The model under review builds one solid part; all positions refer to its coordinate system, in mm. A direction names the side the tool comes from. Coordinates: 2 decimals unless noted, no trailing zeros. Order: outer loops, then holes, each group sorted by start corner. A loop starts at its lowest first (then second) coordinate and runs counter-clockwise, first axis right, second up.
from build123d import *

# Parameters (mm, degrees)
F0_W     = 160
F0_H     = 90
F1_DEPTH = 40
F2_R     = 10
F3_T     = -2.5


with BuildPart() as f1:
    # F0 (on Top) → F1 (new body)
    with BuildSketch(Plane.XY):
        with Locations((-80, -45)):
            Rectangle(F0_W, F0_H)
    extrude(amount=F1_DEPTH)

    # F2
    f2_edges = [f1.edges().sort_by_distance(p)[0] for p in [
        (-160, -90, 20),
        (0, 0, 20),
        (0, -90, 20),
        (-160, 0, 20),
    ]]
    fillet(f2_edges, radius=F2_R)

    # F3
    f3_openings = [f1.faces().sort_by_distance(p)[0] for p in [
        (-80, -45, 40),
    ]]
    offset(amount=F3_T, openings=f3_openings)


solid = f1.part
(1) Tool access review of faces 4 (the face through (-2.85, -3.01, 20.28)), 5 (the face through (-2.5, -45, 21)): name each direction out of +Z, -Z, +X, -X, +Y, -Y from which nothing blocks a thin tool from reaching the whole face with its end or side.
(2) Insertion check: pin 1 Ø10 at (x, y) = (-132.5, -69) entering from +Z. The pin has a flat end and moves straight along its axis. Give the tip position at first contact, or say it passes through.
(3) Consider section A-A (z = 4.5). Give the boundary of the cut face in (x, y), then the cut area to 3 significant figures.
(4) The part is to be moulded in two halves that separate along Y. For faces 1 (the face through (-4.755, -85.361, 21.512)), 2 (the face through (0, -45, 20)), 3 (the face through (-81, -90, 20)), say which applies: +Y half, -Y half, draft (parallel to the pull), parting line (faces both ways), or undercut.
(5) Consider section B-B (x = -97.5). Give the boundary of the cut face in (y, z), then the cut area to 4 significant figures.
(6) Wall thickness on line 1 (X direction, y = -65, z = 29.5); line 2 (Y direction, x = -48, z = 28.5); line 3 (Z direction, x = -30.5, y = -73.5): over which ranges is each line inside the solid? List them lowest first.
(7) Consider section C-C (y = -50). Give the boundary of the cut face in (x, z).
Findings:
1. face 4: +Z, -Z, +X, +Y
1. face 5: +Z
2. pin 1: stops at z = 2.5
3. outline: (-160, -80) arc R10 ccw to (-150, -90) - (-10, -90) arc R10 ccw to (0, -80) - (0, -10) arc R10 ccw to (-10, 0) - (-150, 0) arc R10 ccw to (-160, -10) - close; hole (-157.5, -80) arc R7.5 ccw to (-150, -87.5) - (-10, -87.5) arc R7.5 ccw to (-2.5, -80) - (-2.5, -10) arc R7.5 ccw to (-10, -2.5) - (-150, -2.5) arc R7.5 ccw to (-157.5, -10) - close
3. area: 1,190 mm2
4. face 1: undercut
4. face 2: draft
4. face 3: -Y half
5. outline: (-90, 0) - (0, 0) - (0, 40) - (-2.5, 40) - (-2.5, 2.5) - (-87.5, 2.5) - (-87.5, 40) - (-90, 40) - close
5. area: 412.5 mm2
6. line 1: x = -160 to -157.5, -2.5 to 0
6. line 2: y = -90 to -87.5, -2.5 to 0
6. line 3: z = 0 to 2.5
7. outline: (-160, 0) - (0, 0) - (0, 40) - (-2.5, 40) - (-2.5, 2.5) - (-157.5, 2.5) - (-157.5, 40) - (-160, 40) - close
